```python
from build123d import *

# Parameters (mm, degrees)
CHAMFER1_SIZE = 0.5


with BuildPart() as part:
    # Sketch1 → Revolve1 (revolve)
    with BuildSketch(Plane(origin=(0, 0, 0), x_dir=(0, 0, -1), z_dir=(1, 0, 0))):
        Polygon((-3, 0), (100, 0), (100, 4), (0, 4), (0, 3), (-3, 3), align=None)
    revolve(axis=Axis((0, 0, 3), (0, 0, 1)))

    # Chamfer1
    chamfer1_edges = [part.edges().sort_by_distance(p)[0] for p in [
        (0, -4, -100),
        (0, -3, 3),
    ]]
    chamfer(chamfer1_edges, length=CHAMFER1_SIZE)


solid = part.part
```
CAD build for the part. Positions are in the model's coordinates, mm. A direction names the side the tool comes from. Coordinates: 2 decimals unless noted, no trailing zeros. Write each loop counter-clockwise with the first axis right and the second up, starting at its lowest first coordinate (ties: lowest second). Pieces come first, ordered by that corner, then holes. Notation, with made-up numbers: (62.25, -18) -> (79.25, -18) arc R9 cw to (79.25, -3) -> close; hole circle Ø4 at (-21, 11). An arc over 180 degrees is marked (long way). Use CSV: the item, a comma, the result in double quotes. Start each with the question number.
Item 1: Wall check: probe 1 along Y at (x, z) = (-0.25, -55); probe 2 along Y at (x, z) = (-2.5, -81). Give the ranges that are in metal, low to high.
Item 2: Drop flat-ended pins along their axis: P1, Ø2, axis at y = -2.5, z = -41, coming from the +X side; P2, Ø2, axis at y = -2.5, z = -40.5, coming from the -X side. Give the stop position or say it passes through.
Item 3: Band-saw the part on A-A, the plane z = -83. Write the cut outline in (x, y).
Item 4: Tool access for faces 1 (the flat face through (-3, 1, 0)), 2 (the flat face through (0, 0, -100)): list every direction of +Z, -Z, +X, -X, +Y, -Y with a clear straight run to the whole face (end or side of a thin tool).
Response values:
1,probe 1,"y = -3.99 to 3.99"
1,probe 2,"y = -3.12 to 3.12"
2,P1,"stops at x = 3.71"
2,P2,"stops at x = -3.71"
3,outline,"circle Ø8 at (0, 0)"
4,face 1,"+Z"
4,face 2,"-Z, +X, -X, +Y, -Y"
